Verification items for this drawing (mm, ordinates from the low corner). A direction names the side the tool comes from. Give positions to 0.01 mm unless a question says otherwise; leave off trailing zeros. Loops run counter-clockwise (first coordinate to the right, second up) from the corner with the lowest first, then second, coordinate; pieces in that order, holes last. Notation, with made-up numbers: M 68.25,9.25 L 93.25,9.25 A15 ccw 93.25,38.25 Z; hole C 64.5,45.5 d2. An arc over 180 degrees is marked long. Answer in a Markdown table with one row per item.
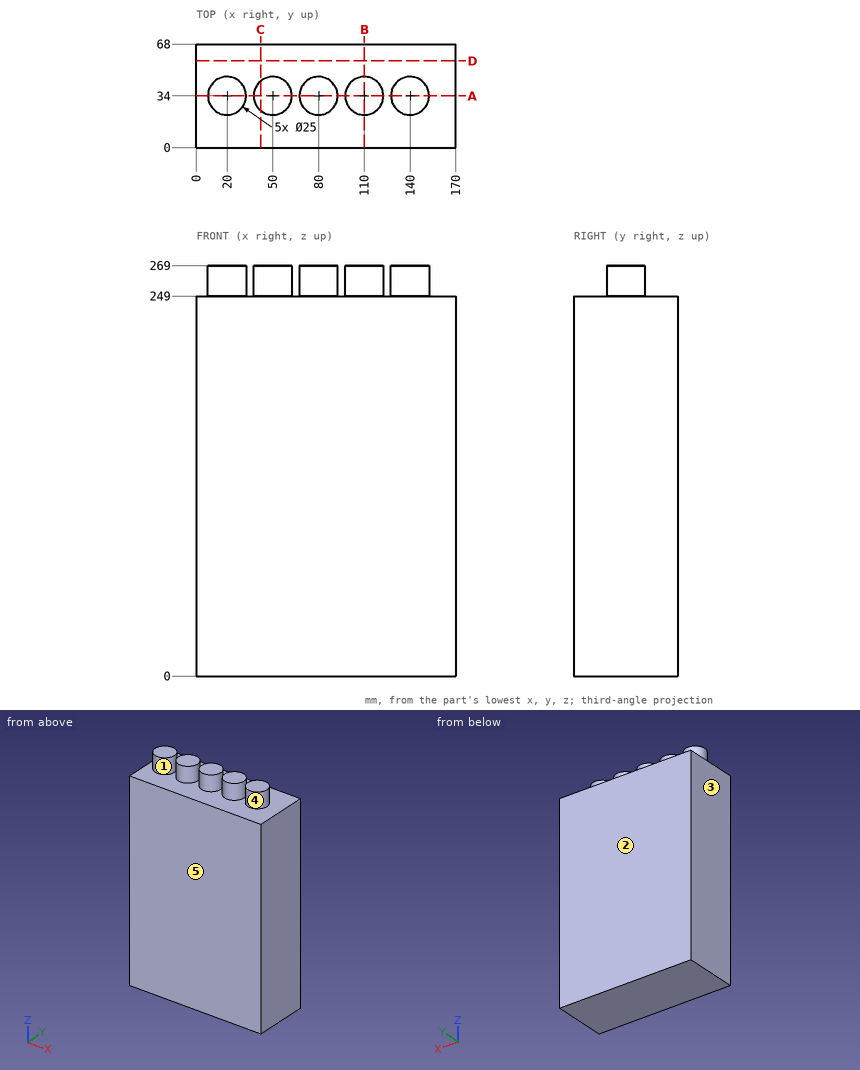
Item 1: Release check for a two-part mould opening along X. For the marked faces 1, 2 and 3 record: released by +X, released by -X, zero draft, split by the parting line, or undercut.
Reported:
| item | result |
|---|---|
| face 1 | undercut |
| face 2 | zero draft |
| face 3 | released by -X |
Item 2: Scan lines: L1, parallel to Z at x = 92.5, y = 15; L2, parallel to Y at x = 119, z = 250. Record each from-to range of solid material in increasing order. Write a range as [from, to].
Reported:
| item | result |
|---|---|
| L1 | z = [0, 249] |
| L2 | y = [25.33, 42.67] |
Item 3: Go/stop test with flat-tipped pins: pin 1 (6 mm diameter, centred on y = 15, z = 214.5, fed in from -X); pin 2 (4 mm diameter, centred on x = 22, y = 15, fed in from +Z). Record where each tip stops, or that it passes through.
Reported:
| item | result |
|---|---|
| pin 1 | stops at x = 0 |
| pin 2 | stops at z = 249 |
Item 4: Sectioned sample at B-B (x = 110). Record the cut outline in (y, z).
Reported:
| item | result |
|---|---|
| outline | M 0,0 L 68,0 L 68,249 L 46.5,249 L 46.5,269 L 21.5,269 L 21.5,249 L 0,249 Z |
Item 5: Tool access check on the marked faces 4 and 5. Record the directions out of +Z, -Z, +X, -X, +Y, -Y that give a thin tool (end or side, any length) a straight path to the whole face; none if there is none.
Reported:
| item | result |
|---|---|
| face 4 | +Z |
| face 5 | +Z, -Z, +X, -X, -Y |
Item 6: Sectioned sample at C-C (x = 42). Record the cut outline in (y, z).
Reported:
| item | result |
|---|---|
| outline | M 0,0 L 68,0 L 68,249 L 43.6,249 L 43.6,269 L 24.4,269 L 24.4,249 L 0,249 Z |
Item 7: Sectioned sample at A-A (y = 34). Record the cut outline in (x, z).
Reported:
| item | result |
|---|---|
| outline | M 0,0 L 170,0 L 170,249 L 152.5,249 L 152.5,269 L 127.5,269 L 127.5,249 L 122.5,249 L 122.5,269 L 97.5,269 L 97.5,249 L 92.5,249 L 92.5,269 L 67.5,269 L 67.5,249 L 62.5,249 L 62.5,269 L 37.5,269 L 37.5,249 L 32.5,249 L 32.5,269 L 7.5,269 L 7.5,249 L 0,249 Z |
Item 8: Sectioned sample at D-D (y = 57). Record the cut outline in (x, z).
Reported:
| item | result |
|---|---|
| outline | M 0,0 L 170,0 L 170,249 L 0,249 Z |
